The listing builds one solid part. Answer for the finished solid, in the listing's coordinates (mm). Coordinates: 2 decimals unless noted, no trailing zeros. Order: outer loops, then holes, each group sorted by start corner. A loop starts at its lowest first (then second) coordinate and runs counter-clockwise, first axis right, second up. Notation, with made-up numbers: (-7.75, 60.25) -> (47.25, 60.25) arc R25 ccw to (47.25, 82.25) -> close; hole circle Ø10 at (40, 19.5). An arc over 180 degrees is marked (long way). Put each result on its own line as item: value. Start each with the question number.
```python
from build123d import *

# Parameters (mm, degrees)
F1_DEPTH = 170
F2_DEPTH = 400
F3_W     = 18.6485039899
F3_H     = 8
F3_W_2   = 19.9612321942
F3_R     = 3.4
F3_R_2   = 2.1
F4_DEPTH = 170
F5_R     = 2


# Not quite as in the source:
# - a pattern or mirror of a feature is missing from the dataset's text; its kind, count and spacing are read off the source's solid


with BuildPart() as f1:
    # F0 (on Front) → F1 (new body)
    with BuildSketch(Plane.XZ):
        Polygon((15, -15), (15, 15), (4, 15), (4, 13), (8.25, 13), (8.25, 9.5), (4.75, 6), (-4.75, 6), (-8.25, 9.5), (-8.25, 13), (-4, 13), (-4, 15), (-15, 15), (-15, -15), align=None)
        Polygon((4, 13), (4, 15), (-4, 15), (-4, 13), (-8.25, 13), (-8.25, 9.5), (-4.75, 6), (4.75, 6), (8.25, 9.5), (8.25, 13), align=None)
    extrude(amount=F1_DEPTH)

    # F0 (on Front) → F2 (cut)
    with BuildSketch(Plane.XZ):
        Polygon((4, 13), (4, 15), (-4, 15), (-4, 13), (-8.25, 13), (-8.25, 9.5), (-4.75, 6), (4.75, 6), (8.25, 9.5), (8.25, 13), align=None)
    f2 = extrude(amount=F2_DEPTH, mode=Mode.SUBTRACT)

    # F2_copies: F2 across plane
    add(f2.mirror(Plane(origin=(0, 0, 0), x_dir=(-1, 0, 0), z_dir=(0, 0, -1))), mode=Mode.SUBTRACT)

    # F3 (on face) → F4 (cut)
    with BuildSketch(Plane(origin=(0, 0, 0), x_dir=(-1, 0, 0), z_dir=(0, 1, 0))):
        Polygon((-6, 4.75), (-9.5, 8.25), (-13, 8.25), (-13, 4), (-13, -4), (-13, -8.25), (-9.5, -8.25), (-6, -4.75), align=None)
        with Locations((-22.3242519949, 0)):
            Rectangle(F3_W, F3_H)
        Polygon((13, 8.25), (9.5, 8.25), (6, 4.75), (6, -4.75), (9.5, -8.25), (13, -8.25), (13, -4), (13, 4), align=None)
        with Locations((22.9806160971, 0)):
            Rectangle(F3_W_2, F3_H)
        Circle(F3_R)
        with Locations((-11.6, 11.6)):
            Circle(F3_R_2)
        with Locations((-11.6, -11.6)):
            Circle(F3_R_2)
        with Locations((11.6, -11.6)):
            Circle(F3_R_2)
        with Locations((11.6, 11.6)):
            Circle(F3_R_2)
    extrude(amount=-F4_DEPTH, mode=Mode.SUBTRACT)

    # F5
    f5_edges = [f1.edges().sort_by_distance(p)[0] for p in [
        (-15, -85, 15),
        (-15, -85, -15),
        (15, -85, -15),
        (15, -85, 15),
    ]]
    fillet(f5_edges, radius=F5_R)


solid = f1.part
```
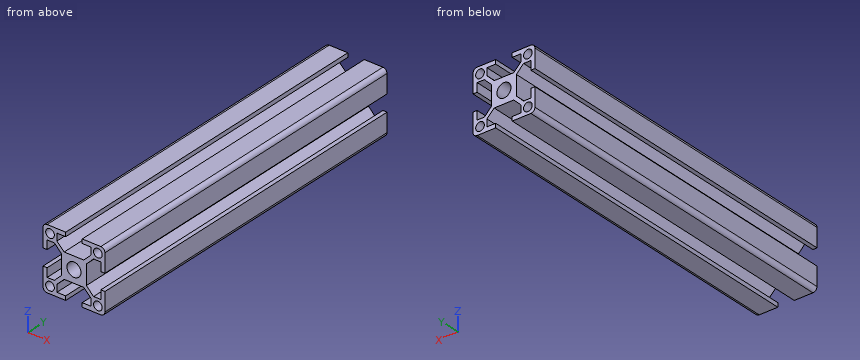
(1) The part is cut by section A-A on z = 0. Determine the outline of the cut face in (x, y).
(2) The part is cut by section B-B on x = 0. Determine the outline of the cut face in (y, z).
(3) The part is cut by section C-C on y = -15. Count the separate pieces of the cut face and the enclosed holes in it, plus the area to 3 significant figures.
(4) Each of these flat-tipped pins is pushed along its axis until it touches: P1, Ø2, axis at x = -1, y = -22, coming from the -Z side; P2, Ø0.6, axis at y = -116.5, z = 14, coming from the -X side; P3, Ø1.5, axis at x = 3, y = -149.5, coming from the +Z side; P4, Ø2.5, axis at x = 11.6, z = 11.6, coming from the +Y side. Where does it stop, or does it pass through?
(5) Find the intervals of material crossed by L1, parallel to Z at x = -11.6, y = -75; L2, parallel to Z at x = 13.5, y = -64.5; L3, parallel to Z at x = 5, y = -151, in increasing order.
Worked out:
1. outline: (-6, -170) -> (-3.4, -170) -> (-3.4, 0) -> (-6, 0) -> close; (3.4, -170) -> (6, -170) -> (6, 0) -> (3.4, 0) -> close
2. outline: (-170, -6) -> (0, -6) -> (0, -3.4) -> (-170, -3.4) -> close; (-170, 3.4) -> (0, 3.4) -> (0, 6) -> (-170, 6) -> close
3. separate pieces: 1
3. enclosed holes: 5
3. area: 328 mm2
4. P1: z = -6
4. P2: x = -14.87
4. P3: z = 6
4. P4: through
5. L1: -15 to -13.7, -9.5 to -8.25, 8.25 to 9.5, 13.7 to 15
5. L2: -14.94 to -12.49, -10.71 to -4, 4 to 10.71, 12.49 to 14.94
5. L3: -15 to -13, -6.25 to 6.25, 13 to 15
